from build123d import *

# Parameters (mm, degrees)
SKETCH1_R           = 13.4
BOSS_EXTRUDE1_DEPTH = 80
FILLET1_R           = 5
FILLET2_R           = 3


with BuildPart() as part:
    # Sketch1 → Boss-Extrude1 (new body)
    with BuildSketch(Plane(origin=(0, 0, 0), x_dir=(1, 0, 0), z_dir=(0, 1, 0))):
        Polygon((-17.4, 17.4), (17.4, 17.4), (82.6, 17.4), (82.6, 13.4), (17.4, 13.4), (17.4, -17.4), (-17.4, -17.4), align=None)
        with Locations(Location((0, 0, 0), (0, 0, 270))):
            Circle(SKETCH1_R, mode=Mode.SUBTRACT)
    boss_extrude1 = extrude(amount=BOSS_EXTRUDE1_DEPTH)

    # Mirror3: Boss-Extrude1 across plane
    add(boss_extrude1.mirror(Plane(origin=(82.6, 80, 0), x_dir=(0, 0, 1), z_dir=(1, 0, 0))))

    # Fillet1
    fillet1_edges = [part.edges().sort_by_distance(p)[0] for p in [
        (17.4, 40, -13.4),
        (-17.4, 40, -17.4),
        (147.8, 40, -13.4),
        (182.6, 40, -17.4),
    ]]
    fillet(fillet1_edges, radius=FILLET1_R)

    # Fillet2
    fillet2_edges = [part.edges().sort_by_distance(p)[0] for p in [
        (17.4, 40, 17.4),
        (-17.4, 40, 17.4),
        (147.8, 40, 17.4),
        (182.6, 40, 17.4),
    ]]
    fillet(fillet2_edges, radius=FILLET2_R)


solid = part.part
The model under review builds one solid part; all positions refer to its coordinate system, in mm. A direction names the side the tool comes from. Round coordinates to 2 decimals unless told otherwise and drop trailing zeros. Loops run counter-clockwise (first coordinate to the right, second up) from the corner with the lowest first, then second, coordinate; pieces in that order, holes last. Notation, with made-up numbers: (19.25, -15) -> (55.25, -15) arc R25 ccw to (55.25, 11) -> close; hole circle Ø6 at (-19.5, 87.25). An arc over 180 degrees is marked (long way). Write item = value, one per line. Start each with the question number.
Item 1: To check wall thickness, follow L1, parallel to X at y = 25, z = 0; L2, parallel to X at y = 24.5, z = 9; L3, parallel to Z at x = 173, y = 65.5. State the ranges of each line that lie inside material, in increasing order.
Item 2: For faces 1 (the cylindrical face through (146.37, 40.56, -11.9)), 2 (the flat face through (82, 0, -14)), list the 3-axis set-ups (+Z, -Z, +X, -X, +Y, -Y) from which the entire face can be reached by the end or side of a thin tool; tool diameter is ignored.
Item 3: Take a section at D-D on x = 114. Give the boundary of the cut face in (y, z), plus the area to 3 significant figures.
Item 4: Take a section at A-A on z = 0. Give the boundary of the cut face in (x, y), plus the area to 3 significant figures.
Item 5: Take a section at C-C on y = 33.5. Give the boundary of the cut face in (x, z).
Item 6: Take a section at B-B on x = 0. Give the boundary of the cut face in (y, z).
Item 7: Insertion check: pin 1 (5 mm diameter, centred on x = 6.5, z = -13, fed in from -Y); pin 2 (8 mm diameter, centred on x = 25, y = 28.5, fed in from +Z); pin 3 (1.5 mm diameter, centred on x = 47, z = -11.5, fed in from +Y). Each pin has a flat end and moves straight along its axis. Give the tip position at first contact, or say it passes through.
Result:
q1.L1 = -17.4 to -13.4, 13.4 to 17.4, 147.8 to 151.8, 178.6 to 182.6
q1.L2 = -17.4 to -9.93, 9.93 to 17.4, 147.8 to 155.27, 175.13 to 182.6
q1.L3 = -17.4 to -10.9, 10.9 to 17.4
q2.face_1 = +Z, +Y, -Y
q2.face_2 = +Z, -Z, +X, -X, -Y
q3.outline = (0, -17.4) -> (80, -17.4) -> (80, -13.4) -> (0, -13.4) -> close
q3.area = 320 mm²
q4.outline = (-17.4, 0) -> (-13.4, 0) -> (-13.4, 80) -> (-17.4, 80) -> close; (13.4, 0) -> (17.4, 0) -> (17.4, 80) -> (13.4, 80) -> close; (147.8, 0) -> (151.8, 0) -> (151.8, 80) -> (147.8, 80) -> close; (178.6, 0) -> (182.6, 0) -> (182.6, 80) -> (178.6, 80) -> close
q4.area = 1,280 mm²
q5.outline = (-17.4, -12.4) arc R5 ccw to (-12.4, -17.4) -> (177.6, -17.4) arc R5 ccw to (182.6, -12.4) -> (182.6, 14.4) arc R3 ccw to (179.6, 17.4) -> (150.8, 17.4) arc R3 ccw to (147.8, 14.4) -> (147.8, -8.4) arc R5 cw to (142.8, -13.4) -> (22.4, -13.4) arc R5 cw to (17.4, -8.4) -> (17.4, 14.4) arc R3 ccw to (14.4, 17.4) -> (-14.4, 17.4) arc R3 ccw to (-17.4, 14.4) -> close; hole circle Ø26.8 at (0, 0); hole circle Ø26.8 at (165.2, 0)
q6.outline = (0, -17.4) -> (80, -17.4) -> (80, -13.4) -> (0, -13.4) -> close; (0, 13.4) -> (80, 13.4) -> (80, 17.4) -> (0, 17.4) -> close
q7.pin_1 = 0
q7.pin_2 = -13.2
q7.pin_3 = through
